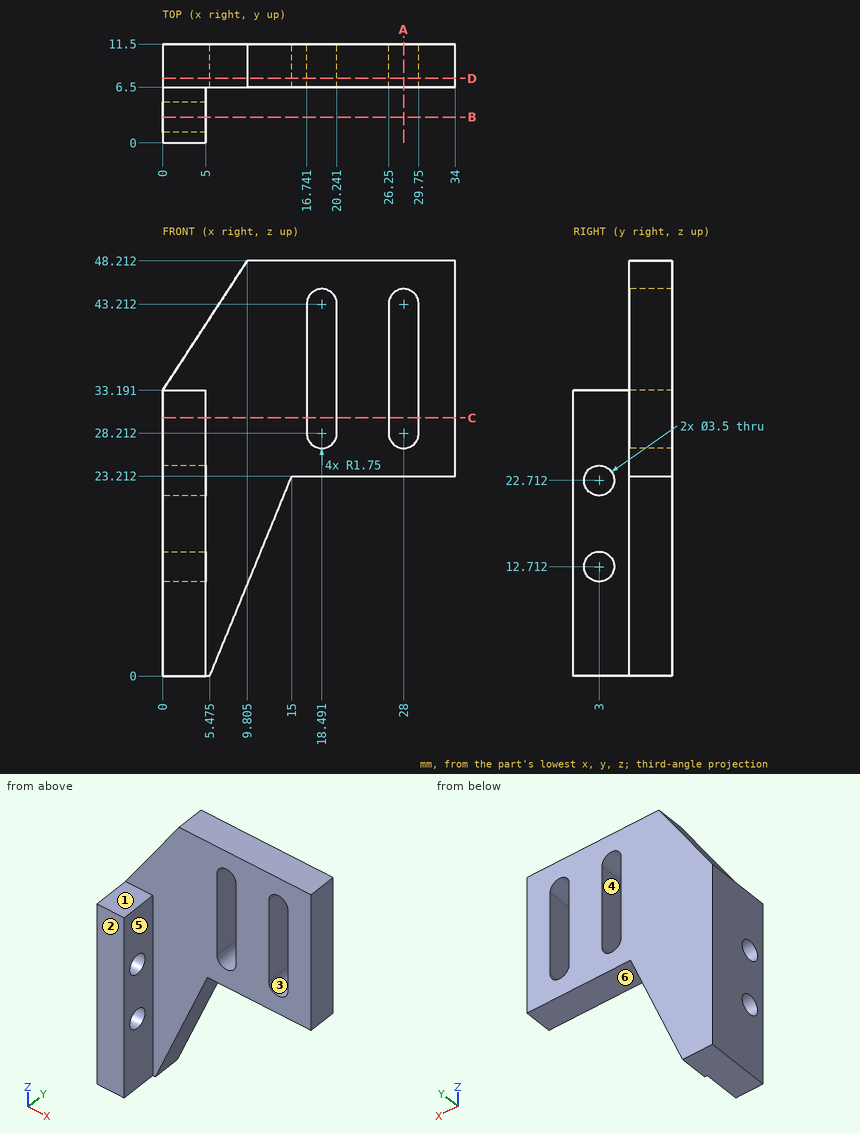
Geometry check sheet. Reference: drawing and pictorial views, mm from the part's lowest x, y, z. A direction names the side the tool comes from. Round coordinates to 2 decimals unless told otherwise and drop trailing zeros. Loops run counter-clockwise (first coordinate to the right, second up) from the corner with the lowest first, then second, coordinate; pieces in that order, holes last.
1. Sectioned sample at C-C on z = 30. Record the boundary of the cut face in (x, y).
2. Set-up check for the marked faces 1, 2 and 3: record each of +Z, -Z, +X, -X, +Y, -Y from which the full face is reachable in a straight line by a thin tool's end or side.
3. Gauge pin test, flat ends, axial feed: pin 1 Ø5.5 at (x, y) = (3.5, 4.5) entering from +Z (1 decimal); pin 2 Ø1.5 at (y, z) = (2, 32) entering from +X; pin 3 Ø5.5 at (x, y) = (24, 9.5) entering from -Z. Record the tip position at first contact, or that the pin passes through.
4. Mould release check, pull along Z, two halves, no side actions. Record for the marked faces 4, 5 and 6: released by +Z, released by -Z, zero draft, split by the parting line, or undercut.
5. Sectioned sample at A-A on x = 28. Record the boundary of the cut face in (y, z), and give its area (3 significant figures).
6. Scan lines: probe 1 along X at (y, z) = (7.5, 32); probe 2 along X at (y, z) = (9.75, 43.5) (1 decimal); probe 3 along Y at (x, z) = (9, 11). Record each from-to range of solid material in increasing order.
7. Sectioned sample at B-B on y = 3. Record the boundary of the cut face in (x, z).
8. Sectioned sample at D-D on y = 7.5. Give the number of separate pieces and of enclosed holes in the cut face, and give its area (3 significant figures).
Recorded:
1. outline: (0, 0) - (5, 0) - (5, 6.5) - (16.74, 6.5) - (16.74, 11.5) - (0, 11.5) - close; (20.24, 6.5) - (26.25, 6.5) - (26.25, 11.5) - (20.24, 11.5) - close; (29.75, 6.5) - (34, 6.5) - (34, 11.5) - (29.75, 11.5) - close
2. face 1: +Z, +X, -X, -Y
2. face 2: +Z, -Z, +X, -X, -Y
2. face 3: +Y, -Y
3. pin 1: stops at z = 41.4
3. pin 2: stops at x = 5
3. pin 3: stops at z = 23.21
4. face 4: undercut
4. face 5: zero draft
4. face 6: released by -Z
5. outline: (6.5, 23.21) - (11.5, 23.21) - (11.5, 26.46) - (6.5, 26.46) - close; (6.5, 44.96) - (11.5, 44.96) - (11.5, 48.21) - (6.5, 48.21) - close
5. area: 32.5 mm2
6. probe 1: x = 0 to 16.74, 20.24 to 26.25, 29.75 to 34
6. probe 2: x = 6.7 to 16.8, 20.2 to 26.3, 29.7 to 34
6. probe 3: y = 6.5 to 11.5
7. outline: (0, 0) - (5, 0) - (5, 10.96) - (0, 10.96) - close; (0, 14.46) - (5, 14.46) - (5, 20.96) - (0, 20.96) - close; (0, 24.46) - (5, 24.46) - (5, 33.19) - (0, 33.19) - close
8. separate pieces: 1
8. enclosed holes: 2
8. area: 890 mm2
